Here's how the part is built. I have some questions about the finished solid (model axes, mm). Face numbers are marked on the shaded views. Round coordinates to 2 decimals unless told otherwise and drop trailing zeros. Loops run counter-clockwise (first coordinate to the right, second up) from the corner with the lowest first, then second, coordinate; pieces in that order, holes last. Notation, with made-up numbers: M -9.75,8.25 L 17.25,8.25 A31 cw 17.25,34.25 Z; hole C -23.5,50.5 d9. An arc over 180 degrees is marked long. Answer as CSV lines item,"result".
```python
from build123d import *

# Parameters (mm, degrees)
F0_R     = 30.3887590566
F1_DEPTH = 25.4


with BuildPart() as f1:
    # F0 (on Front) → F1 (new body)
    with BuildSketch(Plane.XZ):
        with Locations((-41.4496473968, 17.9204754531)):
            Circle(F0_R)
    extrude(amount=F1_DEPTH)

    # F2 (on Front) → F3 (revolve)
    with BuildSketch(Plane.XZ):
        Polygon((58.1389442086, 57.0445582271), (19.5620451123, 57.0445582271), (19.835639745, 29.4114630669), (39.2608866096, 43.6384007335), (58.1389442086, 29.4114630669), align=None)
    revolve(axis=Axis((19.6988424286, 0, 43.228010647), (-0.0099004915, 0, 0.9999509889)))


solid = f1.part
```
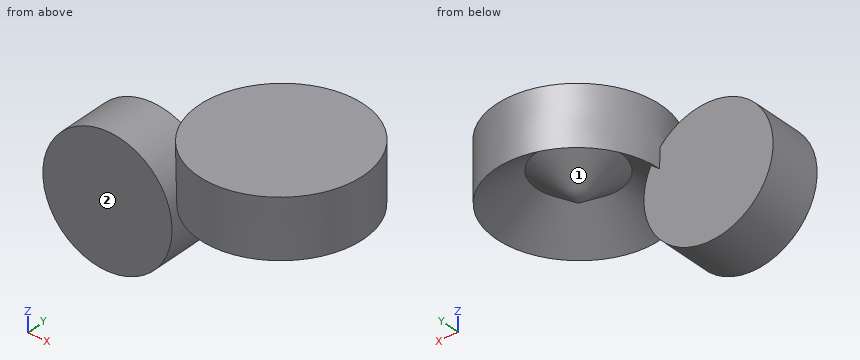
1. We'd pull the mould along X, two halves only. Please class the marked faces 1 and 2: pulls with the +X half, pulls with the -X half, needs draft (parallel to the pull), parting line crosses it, or undercut.
Evaluation:
face 1,"undercut"
face 2,"needs draft"
2. I want a section at A-A, the plane x = -46.5. Please give me the cut outline in (y, z), and give its area (3 significant figures).
Evaluation:
outline,"M -25.4,-12.05 L 0,-12.05 L 0,47.89 L -25.4,47.89 Z"
area,"1,520 mm²"
3. For P1, Ø3, axis at y = -11.5, z = 42.5, coming from the -X side; P2, Ø4, axis at y = -19.5, z = 38.5, coming from the +X side; P3, Ø5, axis at x = -8.5, z = 15.5, coming from the +Y side; P4, Ø18, axis at x = -32, z = 21.5, coming from the +Y side, each with a flat end and sliding along its axis, tell me the tip position at first contact or that it passes through.
Evaluation:
P1,"stops at x = -61.22"
P2,"stops at x = 53.92"
P3,"passes through"
P4,"stops at y = 0"
4. I want a section at B-B, the plane z = 10.5. Please give me the cut outline in (x, y), and give its area (3 significant figures).
Evaluation:
outline,"M -70.92,-25.4 L -11.98,-25.4 L -11.98,0 L -70.92,0 Z"
area,"1,500 mm²"
5. If I drill on line 1 (Y direction, x = -34, z = 38); line 2 (X direction, y = 5, z = 42); line 3 (X direction, y = -19, z = 17.5), over which ranges is the centre line in solid material (lowest first)? Write a range as [from, to].
Evaluation:
line 1,"y = [-25.4, 0]"
line 2,"x = [-18.4, -0.87], [2.64, 36.3], [40.84, 57.81]"
line 3,"x = [-71.84, -11.06]"
